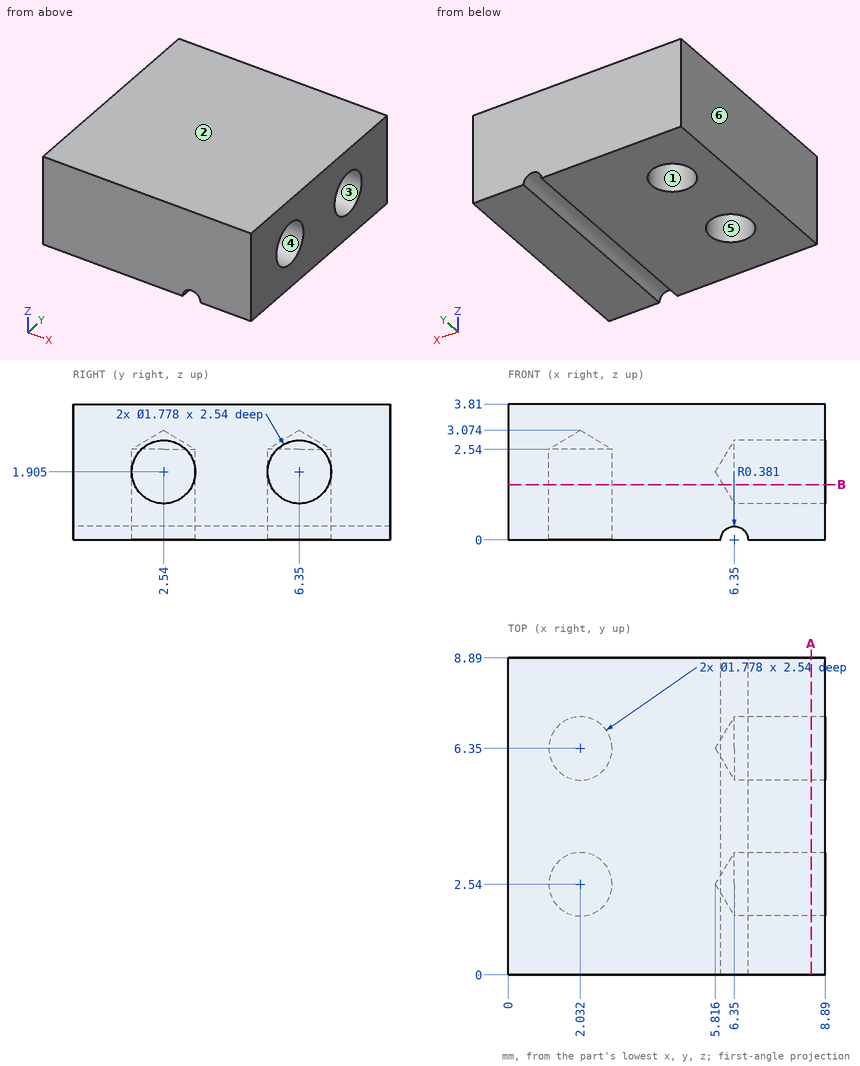
The figure shows three views and two pictorial views of one solid part (mm, origin at its lowest corner). Answer the questions. A direction names the side the tool comes from. Coordinates: 2 decimals unless noted, no trailing zeros. Loops run counter-clockwise (first coordinate to the right, second up) from the corner with the lowest first, then second, coordinate; pieces in that order, holes last. Notation, with made-up numbers: M 61.25,18 L 76.25,18 A18 cw 76.25,48 Z; hole C -24.5,-10.75 d6. An arc over 180 degrees is marked long. Answer as CSV lines item,"result". Start each with the question number.
(1) The part is cut by section B-B (z = 1.55). State how many separate pieces and enclosed holes the cut face has.
(2) For the marked faces 4, 5 and 6, determine the directions among +Z, -Z, +X, -X, +Y, -Y from which every point of the face is accessible in a straight line to the end or side of a thin tool.
(3) Given pin 1 (1.1 mm diameter, centred on x = 2.032, y = 2.54, fed in from -Z); pin 2 (1.6 mm diameter, centred on y = 6.35, z = 1.905, fed in from +X), each flat-ended and moving along its own axis, determine where each tip first touches the part or whether it passes through.
(4) The part is cut by section A-A (x = 8.5). Give the vertices of the cut face in (y, z) (3 decimals).
(5) The mould has two halves that part along Z. Classify the marked faces 1, 2 and 3: pulls with the +Z half, pulls with the -Z half, needs draft (parallel to the pull), parting line crosses it, or undercut.
(6) Find the intervals of material crossed by L1, parallel to Z at x = 7.4, y = 2.54; L2, parallel to Y at x = 1.25, z = 0.5; L3, parallel to Y at x = 7.25, z = 2.4, in increasing order. Write a range as [from, to].
Determined:
1,separate pieces,"1"
1,enclosed holes,"2"
2,face 4,"+X"
2,face 5,"-Z"
2,face 6,"+Z, -Z, -X, +Y, -Y"
3,pin 1,"z = 2.74"
3,pin 2,"x = 6.3"
4,outline,"M 0,0 L 8.89,0 L 8.89,3.81 L 0,3.81 Z; hole C 2.54,1.905 d1.778; hole C 6.35,1.905 d1.778"
5,face 1,"needs draft"
5,face 2,"pulls with the +Z half"
5,face 3,"undercut"
6,L1,"[0, 1.02], [2.79, 3.81]"
6,L2,"[0, 2.12], [2.96, 5.93], [6.77, 8.89]"
6,L3,"[0, 1.8], [3.28, 5.61], [7.09, 8.89]"
